The listing builds one solid part. Answer for the finished solid, in the listing's coordinates (mm). A direction names the side the tool comes from. Round coordinates to 2 decimals unless told otherwise and drop trailing zeros. Loops run counter-clockwise (first coordinate to the right, second up) from the corner with the lowest first, then second, coordinate; pieces in that order, holes last. Notation, with made-up numbers: M 48.25,25 L 54.25,25 A9 ccw 54.25,37 Z; hole C -5.5,-11 d4. An arc over 180 degrees is marked long. Answer as a JSON object with one key per item and string values.
```python
from build123d import *

# Parameters (mm, degrees)
F0_W     = 13
F0_H     = 24
F0_W_2   = 9
F0_H_2   = 20
F1_DEPTH = 10
F0_R     = 0.75
F2_DEPTH = 8
F3_DEPTH = 5


with BuildPart() as f1:
    # F0 (on Top) → F1 (new body)
    with BuildSketch(Plane.XY):
        with Locations((8.4202193944, -4.6071633101)):
            Rectangle(F0_W, F0_H)
        with Locations((8.4202193944, -4.6071633101)):
            Rectangle(F0_W_2, F0_H_2, mode=Mode.SUBTRACT)
    extrude(amount=F1_DEPTH)

    # F0 (on Top) → F2 (join)
    with BuildSketch(Plane.XY):
        with Locations((8.4202193944, -4.6071633101)):
            Rectangle(F0_W, F0_H)
        with Locations((8.4202193944, -4.6071633101)):
            Rectangle(F0_W_2, F0_H_2, mode=Mode.SUBTRACT)
        with Locations((8.4202193944, -4.6071633101)):
            Rectangle(F0_W_2, F0_H_2)
        with Locations((5.4202193944, -13.1071633101)):
            Circle(F0_R, mode=Mode.SUBTRACT)
        with Locations((5.4202193944, -11.0071633101)):
            Circle(F0_R, mode=Mode.SUBTRACT)
        with Locations((7.5202193944, -13.1071633101)):
            Circle(F0_R, mode=Mode.SUBTRACT)
        with Locations((5.4202193944, -8.9071633101)):
            Circle(F0_R, mode=Mode.SUBTRACT)
        with Locations((5.4202193944, 3.8928366899)):
            Circle(F0_R, mode=Mode.SUBTRACT)
        with Locations((11.4202193944, 1.8928366899)):
            Circle(F0_R, mode=Mode.SUBTRACT)
    extrude(amount=F2_DEPTH)

    # F0 (on Top) → F3 (join)
    with BuildSketch(Plane.XY):
        with Locations((8.4202193944, -4.6071633101)):
            Rectangle(F0_W, F0_H)
        with Locations((8.4202193944, -4.6071633101)):
            Rectangle(F0_W_2, F0_H_2, mode=Mode.SUBTRACT)
    extrude(amount=-F3_DEPTH)


solid = f1.part
```
Item 1: Straight lines are drawn through the part: line 1 (Y direction, x = 7.5, z = 4.5); line 2 (X direction, y = -7.5, z = -2.5); line 3 (X direction, y = -13.5, z = 1). For each, find the intervals that lie inside material, in ascending order.
Values follow:
{"line 1": "-16.61 to -13.86, -12.36 to 7.39", "line 2": "1.92 to 3.92, 12.92 to 14.92", "line 3": "1.92 to 4.78, 6.06 to 6.88, 8.16 to 14.92"}
Item 2: The part is cut by section D-D (x = 5.5). Give the vertices of the cut face in (y, z).
Values follow:
{"outline": "M -16.61,-5 L -14.61,-5 L -14.61,0 L -13.85,0 L -13.85,8 L -14.61,8 L -14.61,10 L -16.61,10 Z; M -12.36,0 L -11.75,0 L -11.75,8 L -12.36,8 Z; M -10.26,0 L -9.65,0 L -9.65,8 L -10.26,8 Z; M -8.16,0 L 3.15,0 L 3.15,8 L -8.16,8 Z; M 4.64,0 L 5.39,0 L 5.39,-5 L 7.39,-5 L 7.39,10 L 5.39,10 L 5.39,8 L 4.64,8 Z"}
Item 3: The part is cut by section B-B (y = -4). Give the vertices of the cut face in (x, z).
Values follow:
{"outline": "M 1.92,-5 L 3.92,-5 L 3.92,0 L 12.92,0 L 12.92,-5 L 14.92,-5 L 14.92,10 L 12.92,10 L 12.92,8 L 3.92,8 L 3.92,10 L 1.92,10 Z"}
Item 4: The part is cut by section A-A (x = 11.5). Give the vertices of the cut face in (y, z), then the cut area to 3 significant figures.
Values follow:
{"outline": "M -16.61,-5 L -14.61,-5 L -14.61,0 L 1.15,0 L 1.15,8 L -14.61,8 L -14.61,10 L -16.61,10 Z; M 2.64,0 L 5.39,0 L 5.39,-5 L 7.39,-5 L 7.39,10 L 5.39,10 L 5.39,8 L 2.64,8 Z", "area": "208 mm^2"}
Item 5: The part is cut by section C-C (z = 5.5). Give the vertices of the cut face in (x, y), then the cut area to 3 significant figures.
Values follow:
{"outline": "M 1.92,-16.61 L 14.92,-16.61 L 14.92,7.39 L 1.92,7.39 Z; hole C 5.42,-13.11 d1.5; hole C 5.42,-11.01 d1.5; hole C 5.42,-8.91 d1.5; hole C 5.42,3.89 d1.5; hole C 7.52,-13.11 d1.5; hole C 11.42,1.89 d1.5", "area": "301 mm^2"}
Item 6: Determine the mould class of faces 1 (the face through (1.92, -5, 3)), 2 (the face through (8, -4, 0)), 3 (the face through (14, -4, -5)), 4 (the face through (5.823, 4.525, 3.944)) for opening direction X: released by +X, released by -X, zero draft, split by the parting line, or undercut.
Values follow:
{"face 1": "released by -X", "face 2": "undercut", "face 3": "zero draft", "face 4": "undercut"}
Item 7: Flat-ended cylindrical pins translate along their axes: P1, Ø4.5, axis at x = 8.5, y = -3, coming from the +Z side; P2, Ø2.5, axis at x = 7.52, y = -13.11, coming from the -Z side; P3, Ø0.9, axis at x = 5.42, y = -8.91, coming from the -Z side. Find the tip coordinate at first contact, or state that the pin passes through.
Values follow:
{"P1": "z = 8", "P2": "z = 0", "P3": "through"}
Item 8: Which of the six approach directions +Z, -Z, +X, -X, +Y, -Y give full straight-line access (tool end or side, diameter ignored) to faces 5 (the face through (8, -14.607, -2)), 6 (the face through (3.92, -5, 9)), 7 (the face through (14.92, -5, 3))?
Values follow:
{"face 5": "-Z", "face 6": "+Z", "face 7": "+Z, -Z, +X, +Y, -Y"}
